Here's how the part is built. I have some questions about the finished solid (model axes, mm). Coordinates: 2 decimals unless noted, no trailing zeros. Write each loop counter-clockwise with the first axis right and the second up, starting at its lowest first coordinate (ties: lowest second). Pieces come first, ordered by that corner, then holes.
Item 1: If we mould it in two halves opening along X, with no side actions, what happens to faces 1 (the face through (-83.945, 38.979, 0.986)), 2 (the face through (-3, 0, 1)), 3 (the face through (1, 11, 0))? For each: pulls with the +X half, pulls with the -X half, needs draft (parallel to the pull), parting line crosses it, or undercut.
Item 2: Please list where these lines run through material, in increasing order: line 1 (Y direction, x = -52, z = 1.3); line 2 (X direction, y = -21, z = 0.2); line 3 (X direction, y = -23, z = 1.5).
Item 3: I want a section at D-D (y = -33). Please give me the cut outline in (x, z).
Item 4: I'm going to push a flat-ended pin straight in: P1, Ø1.9, axis at x = 87.5, y = 8, coming from the -Z side. Where does the tip first touch, or does it pass through?
Item 5: I want a section at A-A (y = -12). Please give me the cut outline in (x, z).
Item 6: I want a section at C-C (x = -78.5). Please give me the cut outline in (y, z), and give its area (3 significant figures).
Item 7: I want a section at B-B (z = 0.8). Count the separate pieces of the cut face and the enclosed holes in it, and give its area (3 significant figures).
from build123d import *

# Parameters (mm, degrees)
SKETCH_1_R          = 1.55
SKETCH_1_R_2        = 1.51
SKETCH_1_R_3        = 18
EXTRUDE_1_DEPTH     = 2
SKETCH_2_R          = 1.55
SKETCH_2_R_2        = 3
CUT_EXTRUDE_1_DEPTH = 10


with BuildPart() as part:
    # 草图1 → 凸台-拉伸1 (new body)
    with BuildSketch(Plane.XY):
        with BuildLine():
            Line((-62.5, 48), (62.5, 48))
            ThreePointArc((62.5, 48), (83.713203436, 39.213203436), (92.5, 18))
            Line((92.5, 18), (92.5, -18))
            ThreePointArc((92.5, -18), (83.713203436, -39.213203436), (62.5, -48))
            Line((62.5, -48), (-62.5, -48))
            ThreePointArc((-62.5, -48), (-83.713203436, -39.213203436), (-92.5, -18))
            Line((-92.5, -18), (-92.5, 18))
            ThreePointArc((-92.5, 18), (-83.713203436, 39.213203436), (-62.5, 48))
        make_face()
        with Locations((-64.5, 0)):
            Circle(SKETCH_1_R, mode=Mode.SUBTRACT)
        with Locations((-14.5, 0)):
            Circle(SKETCH_1_R, mode=Mode.SUBTRACT)
        with Locations((14.5, 0)):
            Circle(SKETCH_1_R, mode=Mode.SUBTRACT)
        with Locations((64.5, 0)):
            Circle(SKETCH_1_R, mode=Mode.SUBTRACT)
        with Locations((27, 21.650635095)):
            Circle(SKETCH_1_R, mode=Mode.SUBTRACT)
        with Locations((52, 21.650635095)):
            Circle(SKETCH_1_R, mode=Mode.SUBTRACT)
        with Locations((52, -21.650635095)):
            Circle(SKETCH_1_R, mode=Mode.SUBTRACT)
        with Locations((27, -21.650635095)):
            Circle(SKETCH_1_R, mode=Mode.SUBTRACT)
        with Locations((-52, -21.650635095)):
            Circle(SKETCH_1_R, mode=Mode.SUBTRACT)
        with Locations((-52, 21.650635095)):
            Circle(SKETCH_1_R, mode=Mode.SUBTRACT)
        with Locations((-27, -21.650635095)):
            Circle(SKETCH_1_R_2, mode=Mode.SUBTRACT)
        with Locations((-27, 21.650635095)):
            Circle(SKETCH_1_R, mode=Mode.SUBTRACT)
        with Locations((-39.5, 0)):
            Circle(SKETCH_1_R_3, mode=Mode.SUBTRACT)
        with Locations((39.5, 0)):
            Circle(SKETCH_1_R_3, mode=Mode.SUBTRACT)
        with Locations((57.5, -43)):
            Circle(SKETCH_1_R, mode=Mode.SUBTRACT)
        with Locations((37.5, -43)):
            Circle(SKETCH_1_R, mode=Mode.SUBTRACT)
        with Locations((-57.5, -43)):
            Circle(SKETCH_1_R, mode=Mode.SUBTRACT)
        with Locations((-37.5, -43)):
            Circle(SKETCH_1_R, mode=Mode.SUBTRACT)
        with Locations((-57.5, 43)):
            Circle(SKETCH_1_R, mode=Mode.SUBTRACT)
        with Locations((-37.5, 43)):
            Circle(SKETCH_1_R, mode=Mode.SUBTRACT)
        with Locations((37.5, 43)):
            Circle(SKETCH_1_R, mode=Mode.SUBTRACT)
        with Locations((57.5, 43)):
            Circle(SKETCH_1_R, mode=Mode.SUBTRACT)
        with Locations((15, -43)):
            Circle(SKETCH_1_R, mode=Mode.SUBTRACT)
        with Locations((-5, -43)):
            Circle(SKETCH_1_R, mode=Mode.SUBTRACT)
        with Locations((-5, 43)):
            Circle(SKETCH_1_R, mode=Mode.SUBTRACT)
        with Locations((15, 43)):
            Circle(SKETCH_1_R, mode=Mode.SUBTRACT)
        with Locations((85.596988313, 27.567085809)):
            Circle(SKETCH_1_R, mode=Mode.SUBTRACT)
        with Locations((72.067085809, 41.096988313)):
            Circle(SKETCH_1_R, mode=Mode.SUBTRACT)
        with Locations((72.067085809, -41.096988313)):
            Circle(SKETCH_1_R, mode=Mode.SUBTRACT)
        with Locations((85.596988313, -27.567085809)):
            Circle(SKETCH_1_R, mode=Mode.SUBTRACT)
        with Locations((-85.596988313, -27.567085809)):
            Circle(SKETCH_1_R, mode=Mode.SUBTRACT)
        with Locations((-72.067085809, -41.096988313)):
            Circle(SKETCH_1_R, mode=Mode.SUBTRACT)
        with Locations((-85.596988313, 27.567085809)):
            Circle(SKETCH_1_R, mode=Mode.SUBTRACT)
        with Locations((-72.067085809, 41.096988313)):
            Circle(SKETCH_1_R, mode=Mode.SUBTRACT)
    extrude(amount=EXTRUDE_1_DEPTH)

    # 草图2 → 切除-拉伸1 (cut)
    with BuildSketch(Plane.XY.offset(2)):
        with Locations((87.5, 8)):
            Circle(SKETCH_2_R)
        with Locations((87.5, -2)):
            Circle(SKETCH_2_R)
        with Locations((-87.5, 8)):
            Circle(SKETCH_2_R)
        with Locations((-87.5, -2)):
            Circle(SKETCH_2_R)
        Circle(SKETCH_2_R_2)
    extrude(amount=-CUT_EXTRUDE_1_DEPTH, mode=Mode.SUBTRACT)


solid = part.part
Answer:
1. face 1: pulls with the -X half
1. face 2: undercut
1. face 3: needs draft
2. line 1: y = -48 to -23.2, -20.1 to -12.95, 12.95 to 20.1, 23.2 to 48
2. line 2: x = -92.35 to -53.41, -50.59 to -28.36, -25.64 to 25.59, 28.41 to 50.59, 53.41 to 92.35
2. line 3: x = -92.08 to -52.76, -51.24 to -27.68, -26.32 to 26.24, 27.76 to 51.24, 52.76 to 92.08
3. outline: (-88.48, 0) - (88.48, 0) - (88.48, 2) - (-88.48, 2) - close
4. P1: passes through
5. outline: (-92.5, 0) - (-52.92, 0) - (-52.92, 2) - (-92.5, 2) - close; (-26.08, 0) - (26.08, 0) - (26.08, 2) - (-26.08, 2) - close; (52.92, 0) - (92.5, 0) - (92.5, 2) - (52.92, 2) - close
6. outline: (-43.38, 0) - (43.38, 0) - (43.38, 2) - (-43.38, 2) - close
6. area: 174 mm2
7. separate pieces: 1
7. enclosed holes: 39
7. area: 14,700 mm2
